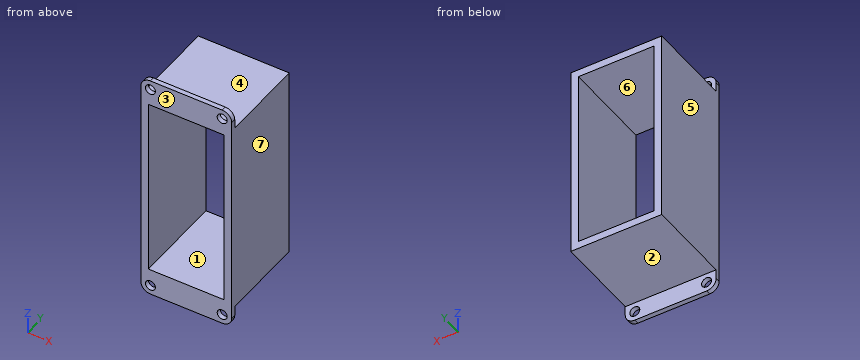
Autodesk Inventor part; units mm, degrees
ref_plane "YZ Plane" through (0, 0, 0) normal (1, 0, 0) x (0, 1, 0)
ref_plane "XZ Plane" through (0, 0, 0) normal (0, 1, 0) x (-1, 0, 0)
ref_plane "XY Plane" through (0, 0, 0) normal (0, 0, 1) x (1, 0, 0)
sketch "Sketch1" plane through (0, 0, 0) normal (0, 1, 0) x (-1, 0, 0)
  line L0 (0, 0) -> (-31.75, 0)
  line L1 (-31.75, 0) -> (-31.75, -76.2)
  line L2 (-31.75, -76.2) -> (0, -76.2)
  line L3 (0, -76.2) -> (0, 0)
  line L4 (-34.925, -79.375) -> (-34.925, 3.175)
  line L5 (-34.925, 3.175) -> (3.175, 3.175)
  line L6 (3.175, 3.175) -> (3.175, -79.375)
  line L7 (3.175, -79.375) -> (-34.925, -79.375)
  dimension "d0" = 31.75
  dimension "d1" = 76.2
  dimension "d2" = 3.175
extrude "Extrusion1" add sketch "Sketch1" along normal blind 38.1
sketch "Sketch2" plane through (-3.175, 0, 3.175) normal (0, 0, 1) x (1, 0, 0)
  line L0 (38.1, 0) -> (38.1, 38.1)
  line L1 (0, 0) -> (38.1, 0)
  line L2 (38.1, 0) -> (38.1, 2)
  line L3 (38.1, 2) -> (0, 2)
  line L4 (0, 2) -> (0, 0)
  point P0 (3.175, 0)
  dimension "d5" = 2
extrude "Extrusion2" add sketch "Sketch2" along normal blind 8
fillet "Fillet1" radius 4 2 edges at (34.925, 1, 11.175) (-3.175, 1, 11.175)
sketch "Sketch3" plane through (-3.175, 2, 3.175) normal (0, 1, 0) x (1, 0, 0)
  arc A0 (0, -4) -> (4, -8) centre (4, -4) ccw
  circle A1 centre (4, -4) radius 2.1
  arc A2 (34.1, -8) -> (38.1, -4) centre (34.1, -4) ccw
  circle A3 centre (34.1, -4) radius 2.1
  point P0 (3.175, 3.175)
  dimension "d9" = 4.2
  dimension "d10" = 4.2
extrude "Extrusion3" cut sketch "Sketch3" against normal blind 8
sketch "Sketch4" plane through (34.925, 0, -79.375) normal (0, 0, -1) x (-1, 0, 0)
  line L0 (38.1, 2) -> (38.1, 0)
  line L1 (0, 0) -> (38.1, 0)
  line L2 (38.1, 0) -> (38.1, 2)
  line L3 (38.1, 2) -> (0, 2)
  line L4 (0, 2) -> (0, 0)
  point P0 (34.925, 0)
  dimension "d13" = 2
extrude "Extrusion4" add sketch "Sketch4" along normal blind 8
fillet "Fillet2" radius 4 2 edges at (34.925, 1, -87.375) (-3.175, 1, -87.375)
sketch "Sketch5" plane through (-3.175, 2, -79.375) normal (0, 1, 0) x (1, 0, 0)
  arc A0 (38.1, 4) -> (34.1, 8) centre (34.1, 4) ccw
  circle A1 centre (34.1, 4) radius 2.1
  arc A2 (4, 8) -> (0, 4) centre (4, 4) ccw
  circle A3 centre (4, 4) radius 2.1
  line L0 (4, 4) -> (0, 4)
  point P0 (3.175, -79.375)
  dimension "d17" = 4.2
  dimension "d18" = 4.2
extrude "Extrusion5" cut sketch "Sketch5" against normal blind 8
properties part number "BatteryHolder"
For this review, take the finished solid that the model builds, in its own axes (mm). Face numbers are marked on the shaded views. A direction names the side the tool comes from. Coordinates: 2 decimals unless noted, no trailing zeros. Order: outer loops, then holes, each group sorted by start corner. A loop starts at its lowest first (then second) coordinate and runs counter-clockwise, first axis right, second up. Notation, with made-up numbers: (-12, 75) -> (18, 75) arc R13 ccw to (18, 89) -> close; hole circle Ø6 at (45, 81.25). An arc over 180 degrees is marked (long way). Use CSV: the item, a comma, the result in double quotes. Start each with the question number.
Item 1: Insertion check: pin 1 (18 mm diameter, centred on x = 23, y = 13, fed in from +Z) (3 decimals); pin 2 (5 mm diameter, centred on x = 0.825, z = 7.175, fed in from +Y); pin 3 (9.5 mm diameter, centred on x = 11.5, y = 16, fed in from -Z) (3 decimals). Each pin has a flat end and moves straight along its axis. Give the tip position at first contact, or say it passes through.
Item 2: We need section C-C, the plane x = 4.5. Give the boundary of the cut face in (y, z) (3 decimals).
Item 3: Draft analysis for pull direction X (two halves, no side actions). For the marked faces 5, 6 and 7, state which applies: pulls with the +X half, pulls with the -X half, needs draft (parallel to the pull), parting line crosses it, or undercut.
Item 4: We need section B-B, the plane y = 9. Give the boundary of the cut face in (x, z) (3 decimals), then the cut area to 3 significant figures.
Item 5: We need section A-A, the plane z = -14. Give the boundary of the cut face in (x, y) (3 decimals), then the cut area to 3 significant figures.
Item 6: Wall thickness on probe 1 along Z at (x, y) = (15, 12) (3 decimals); probe 2 along X at (y, z) = (12.5, -19) (3 decimals); probe 3 along Z at (x, y) = (-0.5, 21.5) (3 decimals): over which ranges is each line inside the solid? List them lowest first.
Item 7: For the marked faces 1, 2, 3 and 4, list the 3-axis set-ups (+Z, -Z, +X, -X, +Y, -Y) from which the entire face can be reached by the end or side of a thin tool; tool diameter is ignored.
Derived:
1,pin 1,"stops at z = 3.175"
1,pin 2,"stops at y = 2"
1,pin 3,"stops at z = -79.375"
2,outline,"(0, -87.375) -> (2, -87.375) -> (2, -79.375) -> (38.1, -79.375) -> (38.1, -76.2) -> (0, -76.2) -> close; (0, 0) -> (38.1, 0) -> (38.1, 3.175) -> (2, 3.175) -> (2, 11.175) -> (0, 11.175) -> close"
3,face 5,"pulls with the -X half"
3,face 6,"undercut"
3,face 7,"pulls with the +X half"
4,outline,"(-3.175, -79.375) -> (34.925, -79.375) -> (34.925, 3.175) -> (-3.175, 3.175) -> close; hole (0, -76.2) -> (31.75, -76.2) -> (31.75, 0) -> (0, 0) -> close"
4,area,"726 mm^2"
5,outline,"(-3.175, 0) -> (0, 0) -> (0, 38.1) -> (-3.175, 38.1) -> close; (31.75, 0) -> (34.925, 0) -> (34.925, 38.1) -> (31.75, 38.1) -> close"
5,area,"242 mm^2"
6,probe 1,"z = -79.375 to -76.2, 0 to 3.175"
6,probe 2,"x = -3.175 to 0, 31.75 to 34.925"
6,probe 3,"z = -79.375 to 3.175"
7,face 1,"+Y, -Y"
7,face 2,"-Z, +X, -X, +Y"
7,face 3,"+Z, -Z, +X, -X, -Y"
7,face 4,"+Z, +X, -X, +Y"
